Can you work these out from the model? Positions are in its coordinate system, mm. Coordinates: 2 decimals unless noted, no trailing zeros. Order: outer loops, then holes, each group sorted by start corner. A loop starts at its lowest first (then second) coordinate and runs counter-clockwise, first axis right, second up. Notation, with made-up numbers: (-23.5, 82) -> (25.5, 82) arc R11 ccw to (25.5, 94) -> close; hole circle Ø9 at (-1.75, 86). An arc over 180 degrees is marked (long way). Return JSON: item names as keys, results as strings. Group by question number.
1) For pin 1 (0.9 mm diameter, centred on y = -123, z = 2, fed in from -X); pin 2 (0.9 mm diameter, centred on x = 128, z = 2.5, fed in from -Y); pin 3 (1.6 mm diameter, centred on x = -132.5, z = 1, fed in from -Y), each with a flat end and sliding along its axis, tell me the tip position at first contact or that it passes through.
2) If I drill on probe 1 along X at (y, z) = (96, 2.5); probe 2 along Y at (x, z) = (62.75, 2.1); probe 3 along X at (y, z) = (65, 2.05), over which ranges is the centre line in solid material (lowest first)? Write a range as from..to.
3) If we section it at A-A, the plane y = 120.5: Please give me the cut outline in (x, z), then the cut area to 3 significant figures.
4) If we section it at B-B, the plane z = 0.85: Please give me the cut outline in (x, y), then the cut area to 3 significant figures.
5) If we section it at C-C, the plane y = -93: Please give me the cut outline in (x, z), then the cut area to 3 significant figures.
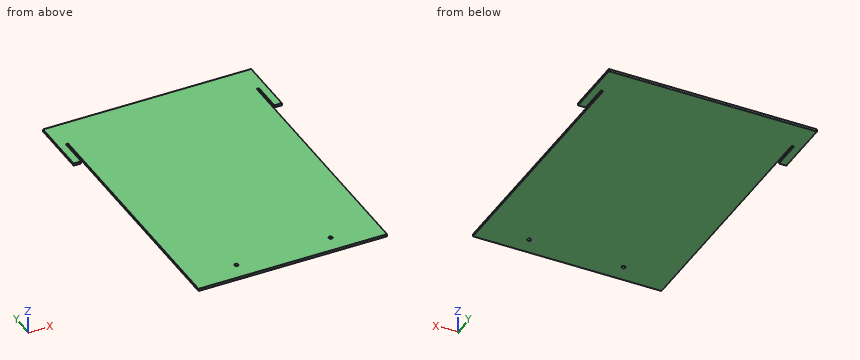
Autodesk Inventor part; units mm, degrees
ref_plane "YZ Plane" through (0, 0, 0) normal (1, 0, 0) x (0, 1, 0)
ref_plane "XZ Plane" through (0, 0, 0) normal (0, 1, 0) x (-1, 0, 0)
ref_plane "XY Plane" through (0, 0, 0) normal (0, 0, 1) x (1, 0, 0)
sketch "Sketch1" plane through (0, 0, 0) normal (0, 0, 1) x (1, 0, 0)
  line L0 (125.5, -166.1125) -> (-125.5, -166.1125)
  line L1 (-125.5, -166.1125) -> (-125.5, 166.1125)
  line L2 (-125.5, 166.1125) -> (125.5, 166.1125)
  line L3 (125.5, 166.1125) -> (125.5, -166.1125)
  line L4 (125.5, -166.1125) -> (-125.5, 166.1125) construction
  line L5 (-125.5, -166.1125) -> (125.5, 166.1125) construction
  line L6 (-125.5, -166.1125) -> (125.5, -166.1125)
  line L7 (125.5, -166.1125) -> (125.5, -214.1125)
  line L8 (125.5, -214.1125) -> (-125.5, -214.1125)
  line L9 (-125.5, -214.1125) -> (-125.5, -166.1125)
  point P0 (0, 0)
  dimension "d0" = 251
  dimension "d1" = 332.225
  dimension "d4" = 48
  dimension "d5" = 0
  dimension "d6" = 0
extrude "Extrusion1" add sketch "Sketch1" along normal blind 3.15
sketch "Sketch2" plane through (0, 0, 3.15) normal (0, 0, 1) x (1, 0, 0)
  line L0 (125.5, 166.1125) -> (-125.5, 166.1125)
  line L1 (-125.5, 166.1125) -> (-138.65, 166.1125)
  line L2 (-138.65, 166.1125) -> (-138.65, 86.1125)
  line L3 (-138.65, 86.1125) -> (-125.5, 86.1125)
  line L4 (-125.5, 86.1125) -> (-125.5, 166.1125)
  line L5 (-125.5, 86.1125) -> (-128.65, 86.1125)
  line L6 (-128.65, 86.1125) -> (-128.65, 126.1125)
  line L7 (-128.65, 126.1125) -> (-125.5, 126.1125)
  line L8 (-125.5, 126.1125) -> (-125.5, 86.1125)
  line L9 (0, 166.1125) -> (0, 0)
  line L10 (125.5, 166.1125) -> (138.65, 166.1125)
  line L11 (138.65, 166.1125) -> (138.65, 86.1125)
  line L12 (138.65, 86.1125) -> (125.5, 86.1125)
  line L13 (125.5, 86.1125) -> (125.5, 166.1125)
  line L14 (125.5, 86.1125) -> (128.65, 86.1125)
  line L15 (128.65, 86.1125) -> (128.65, 126.1125)
  line L16 (128.65, 126.1125) -> (125.5, 126.1125)
  line L17 (125.5, 126.1125) -> (125.5, 86.1125)
  dimension "d7" = 80
  dimension "d8" = 13.15
  dimension "d9" = 3.15
  dimension "d10" = 40
extrude "Extrusion2" add sketch "Sketch2" against normal blind 3.15 contours L4 L7 L6 L3 L2 L1 | L10 L11 L12 L15 L16 L13
sketch "Sketch3" plane through (0, 0, 3.15) normal (0, 0, 1) x (1, 0, 0)
  line L0 (-125.5, -214.1125) -> (125.5, -214.1125)
  circle A0 centre (-62.75, -190.1125) radius 2.5
  line L1 (0, 0) -> (0, -214.1125)
  circle A1 centre (62.75, -190.1125) radius 2.5
  dimension "d13" = 5
  dimension "d14" = 24
  dimension "d15" = 62.75
extrude "Extrusion3" cut sketch "Sketch3" against normal blind 10
equation "\"d0\" = door_x"
equation "\"d1\" = door_z"
equation "\"d4\" = door_overlap"
equation "\"d2\" = clear_acrylic"
equation "\"d7\" = protection_slot_length"
equation "\"d8\" = protection_slot_width + clear_acrylic"
equation "\"d9\" = clear_acrylic"
equation "\"d10\" = 0.5 * protection_slot_length"
equation "\"d11\" = clear_acrylic"
equation "\"d13\" = m5_diameter"
equation "\"d14\" = 0.5 * door_overlap"
equation "\"d15\" = 0.25 * tray_x"
equation "\"sm_thickness\" = 1.5875"
equation "\"very_thick_acrylic\" = 9.45"
equation "\"thick_acrylic\" = 5.88"
equation "\"thin_acrylic\" = 3.15"
equation "\"clear_acrylic\" = 3.15"
equation "\"wood_thickness\" = 6.72"
equation "\"m3_diameter\" = 3"
equation "\"m4_diameter\" = 4"
equation "\"m5_diameter\" = 5"
equation "\"brass_insert_drill\" = 4"
equation "\"m5_brass_insert_drill\" = 6.7"
equation "\"m3_main_length\" = 14"
equation "\"m3_main_nut_width\" = 5.7"
equation "\"m3_main_nut_thickness\" = 2.5"
equation "\"m3_main_extra\" = 1"
equation "\"stepper_screw_space\" = 35"
equation "\"stepper_shaft_diameter\" = 5"
equation "\"stepper_body_diameter\" = 28"
equation "\"laser_body_diameter\" = 12"
equation "\"carrier_y\" = 251"
equation "\"carrier_z\" = 12"
equation "\"visor_x\" = 253.925"
equation "\"visor_y\" = 85.6"
equation "\"protection_slot\" = 44.2"
equation "\"protection_slot_offset\" = 55.25"
equation "\"protection_slot_length\" = 80"
equation "\"window_z\" = 332.225"
equation "\"window_y\" = 93.75"
equation "\"window_overlap\" = 48"
equation "\"door_x\" = 251"
equation "\"door_z\" = 332.225"
equation "\"door_sensor\" = 35"
equation "\"reservoir_x\" = 201"
equation "\"reservoir_y\" = 201"
equation "\"linear_bearing_spacing\" = 271"
equation "\"motor_spacing\" = 337"
equation "\"tray_border\" = 25"
equation "\"tray_x\" = 251"
equation "\"tray_y\" = 251"
equation "\"bed_z\" = 25"
equation "\"crane_z2\" = 12"
equation "\"end_stop_spacing\" = 19"
equation "\"door_overlap\" = 48"
equation "\"acrylic_into_frame\" = 5"
equation "\"protection_slot_width\" = 10"
equation "\"frame_top_z\" = 385"
equation "\"nema17_x\" = 43"
equation "\"drawer_z_from_bottom\" = 25"
equation "\"laser_diameter\" = 12"
equation "\"t_galvo_frame\" = 6.72"
equation "\"laser_z\" = 75"
equation "\"drawer_y\" = 90.3375"
equation "\"laser_y\" = 15"
equation "\"subframe_x\" = 66"
equation "\"galvo_frame_z\" = 85"
equation "\"subframe_y_offset\" = 27.5"
equation "\"drawer_x\" = 257.3"
equation "\"printer_z\" = 289"
equation "\"lcd_x\" = 72"
equation "\"frame_tilt\" = 1deg"
equation "\"frame_foot_z\" = 12"
equation "\"frame_border\" = 48.0375"
equation "\"frame_bottom_z\" = 275"
equation "\"z_min_from_center\" = 115"
equation "\"thumb_nut_diameter\" = 7"
equation "\"laser_z_offset\" = 55"
equation "\"laser_y_offset\" = 19.4"
equation "\"thumb_nut_offset_y\" = 0"
equation "\"galvo_frame_y_offset\" = 27.5"
equation "\"frame_total_z\" = 661.5875"
equation "\"galvo_frame_x\" = 66"
equation "\"drawer_z\" = 278.175"
equation "\"lcd_y\" = 25"
equation "\"m3_press_nut_drill\" = 4.5"
equation "\"m3_head\" = 6"
equation "\"m5_head\" = 10.3"
equation "\"m5_press_nut_drill\" = 6.5"
equation "\"drawer_support_from_top\" = 48"
equation "\"laser_gap\" = 1"
equation "\"frame_screw_from_center\" = 25"
equation "\"drawer_screw_from_center\" = 55"
equation "\"frame_face_y\" = 45"
equation "\"switch_spacing\" = 19"
equation "\"subframe_y\" = 55"
equation "\"al_thickness\" = 1.5875"
equation "\"rivet_diameter\" = 3.3"
equation "\"bend_factor\" = 2.26205"
equation "\"al_bend\" = 3.591"
equation "\"sm_bend\" = 3.591"
equation "\"frame_x\" = 353.375"
equation "\"carrier_z2\" = 25"
equation "\"carrier_y2\" = 76.825"
properties part number "door"
Result sheet:
{
 "1": {"pin 1": "stops at x = -125.5", "pin 2": "stops at y = 126.11", "pin 3": "stops at y = 86.11"},
 "2": {"probe 1": "x = -138.65..-128.65, -125.5..125.5, 128.65..138.65", "probe 2": "y = -214.11..-192.61, -187.61..166.11", "probe 3": "x = -125.5..125.5"},
 "3": {"outline": "(-138.65, 0) -> (-128.65, 0) -> (-128.65, 3.15) -> (-138.65, 3.15) -> close; (-125.5, 0) -> (125.5, 0) -> (125.5, 3.15) -> (-125.5, 3.15) -> close; (128.65, 0) -> (138.65, 0) -> (138.65, 3.15) -> (128.65, 3.15) -> close", "area": "854 mm2"},
 "4": {"outline": "(-138.65, 86.11) -> (-128.65, 86.11) -> (-128.65, 126.11) -> (-125.5, 126.11) -> (-125.5, -214.11) -> (125.5, -214.11) -> (125.5, 126.11) -> (128.65, 126.11) -> (128.65, 86.11) -> (138.65, 86.11) -> (138.65, 166.11) -> (-138.65, 166.11) -> close; hole circle Ø5 at (-62.75, -190.11); hole circle Ø5 at (62.75, -190.11)", "area": "97,200 mm2"},
 "5": {"outline": "(-125.5, 0) -> (125.5, 0) -> (125.5, 3.15) -> (-125.5, 3.15) -> close", "area": "791 mm2"}
}
